from build123d import *

# Parameters (mm, degrees)
SKETCH1_W           = 12
SKETCH1_H           = 600
BOSS_EXTRUDE1_DEPTH = 8
CUT_EXTRUDE1_DEPTH  = 601.083327547
SKETCH3_R           = 3
CUT_EXTRUDE2_DEPTH  = 4.5
SKETCH4_R           = 1.75
CUT_EXTRUDE3_DEPTH  = 601.046873169
LPATTERN1_COUNT     = 24
LPATTERN1_PITCH     = 25


with BuildPart() as part:
    # Sketch1 → Boss-Extrude1 (new body)
    with BuildSketch(Plane.XY):
        with Locations((0, 300)):
            Rectangle(SKETCH1_W, SKETCH1_H)
    extrude(amount=BOSS_EXTRUDE1_DEPTH)

    # Sketch2 → Cut-Extrude1 (cut, through all)
    with BuildSketch(Plane(origin=(0, 600, 0), x_dir=(1, 0, 0), z_dir=(0, 1, 0))):
        with BuildLine():
            Line((-5.5, 0), (-6, -0.5))
            Line((-6, -0.5), (-6, -3.5))
            ThreePointArc((-6, -3.5), (-5.867156742, -4.117156742), (-5.492156742, -4.625))
            ThreePointArc((-5.492156742, -4.625), (-5.322875656, -5), (-5.492156742, -5.375))
            ThreePointArc((-5.492156742, -5.375), (-5.90312152, -7.030330086), (-4.5, -8))
            Line((-4.5, -8), (-7.760322007, -8))
            Line((-7.760322007, -8), (-7.760322007, 0))
            Line((-7.760322007, 0), (-5.5, 0))
        make_face()
        with BuildLine():
            Line((6, -0.5), (6, -3.5))
            ThreePointArc((6, -3.5), (5.867156742, -4.117156742), (5.492156742, -4.625))
            ThreePointArc((5.492156742, -4.625), (5.322875656, -5), (5.492156742, -5.375))
            ThreePointArc((5.492156742, -5.375), (5.90312152, -7.030330086), (4.5, -8))
            Line((4.5, -8), (7.760322007, -8))
            Line((7.760322007, -8), (7.760322007, 0))
            Line((7.760322007, 0), (5.5, 0))
            Line((5.5, 0), (6, -0.5))
        make_face()
    extrude(amount=-CUT_EXTRUDE1_DEPTH, mode=Mode.SUBTRACT)

    # Sketch3 → Cut-Extrude2 (cut)
    with BuildSketch(Plane.XY.offset(8)):
        with Locations((0, 590)):
            Circle(SKETCH3_R)
    cut_extrude2 = extrude(amount=-CUT_EXTRUDE2_DEPTH, mode=Mode.SUBTRACT)

    # Sketch4 → Cut-Extrude3 (cut, through all)
    with BuildSketch(Plane.XY.offset(3.5)):
        with Locations((0, 590)):
            Circle(SKETCH4_R)
    cut_extrude3 = extrude(amount=-CUT_EXTRUDE3_DEPTH, mode=Mode.SUBTRACT)

    # LPattern1: Cut-Extrude2, Cut-Extrude3 ×24
    with Locations(*[(0, -i * LPATTERN1_PITCH, 0) for i in range(1, LPATTERN1_COUNT)]):
        add(cut_extrude2, mode=Mode.SUBTRACT)
        add(cut_extrude3, mode=Mode.SUBTRACT)


solid = part.part
Part model, mm, in its own coordinate system. Give positions to 0.01 mm unless a question says otherwise; leave off trailing zeros. Order: outer loops, then holes, each group sorted by start corner. A loop starts at its lowest first (then second) coordinate and runs counter-clockwise, first axis right, second up. Notation, with made-up numbers: (79, 54.25) -> (118, 54.25) arc R9 ccw to (118, 69.25) -> close; hole circle Ø11 at (-29.75, -20.5). An arc over 180 degrees is marked (long way). Use one line per item in the form item = value.
(1) Saw through at B-B (z = 6.75). Count the separate pieces of the cut face and the enclosed holes in it, then the cut area to 3 significant figures.
Solution:
separate_pieces = 1
enclosed_holes = 24
area = 6,500 mm²
(2) Flat gauge pins, fed straight in: P1, Ø1, axis at y = 107.5, z = 4.5, coming from the -X side; P2, Ø4, axis at x = 0, y = 190, coming from the +Z side; P3, Ø3, axis at x = 0, y = 265, coming from the -Z side; P4, Ø2, axis at y = 164.5, z = 5, coming from the +X side. Where does each tip first touch, or does it go through?
Solution:
P1 = -5.91
P2 = 3.5
P3 = through
P4 = 5.91
(3) Saw through at A-A (y = 49.5). Write the cut outline in (x, z) (3 decimals).
Solution:
outline = (-6, 0.5) -> (-5.5, 0) -> (5.5, 0) -> (6, 0.5) -> (6, 3.5) arc R1.5 ccw to (5.492, 4.625) arc R0.5 cw to (5.492, 5.375) arc R1.5 ccw to (4.5, 8) -> (-4.5, 8) arc R1.5 ccw to (-5.492, 5.375) arc R0.5 cw to (-5.492, 4.625) arc R1.5 ccw to (-6, 3.5) -> close
(4) Drill centre lines: line 1 (X direction, y = 115, z = 6.9); line 2 (X direction, y = 340, z = 3); line 3 (Z direction, x = -4.75, y = 54). Where is each one in solid material? Low to high. Write a range as from..to.
Solution:
line_1 = -5.95..-3, 3..5.95
line_2 = -6..-1.75, 1.75..6
line_3 = 0..7.98
